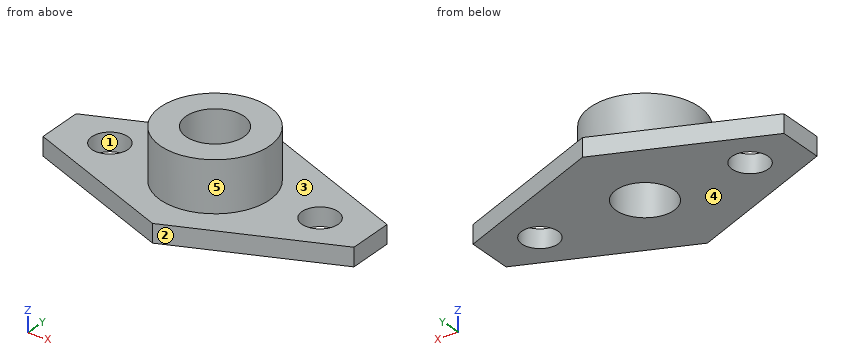
```python
from build123d import *

# Parameters (mm, degrees)
BOSS_EXTRUDE1_DEPTH     = 2.54
SKETCH1_4_R             = 7.560754729
BOSS_EXTRUDE2_DEPTH     = 9.525
CUT_EXTRUDE1_DEPTH      = 27.400295926
CUT_EXTRUDE1_DEPTH_BACK = 9.525
SKETCH1_8_R             = 4
SKETCH1_8_R_2           = 2.5


with BuildPart() as part:
    # Sketch1 → Boss-Extrude1 (new body)
    with BuildSketch(Plane.XY):
        Polygon((-21.5, 3.175), (0, 12), (21.5, 3.175), (21.5, 0), (21.5, -3.175), (0, -12), (-21.5, -3.175), align=None)
    extrude(amount=BOSS_EXTRUDE1_DEPTH)

    # Sketch1_4 → Boss-Extrude2 (add)
    with BuildSketch(Plane.XY):
        with Locations(Location((0, 0, 0), (0, 0, 180))):
            Circle(SKETCH1_4_R)
    extrude(amount=BOSS_EXTRUDE2_DEPTH)

    # Sketch1_8 → Cut-Extrude1 (cut, two sides: drawn at the far end of the back side and taken through both)
    with BuildSketch(Plane.XY.offset(-CUT_EXTRUDE1_DEPTH_BACK)):
        with Locations(Location((0, 0, 0), (0, 0, 180))):
            Circle(SKETCH1_8_R)
        with Locations(Location((14.530377365, 0, 0), (0, 0, 180))):
            Circle(SKETCH1_8_R_2)
        with Locations(Location((-14.530377365, 0, 0), (0, 0, 180))):
            Circle(SKETCH1_8_R_2)
    extrude(amount=CUT_EXTRUDE1_DEPTH + CUT_EXTRUDE1_DEPTH_BACK, mode=Mode.SUBTRACT)


solid = part.part
```
Input: part model. Units: mm. Frame: model coordinates. Face numbers are marked on the shaded views. A direction names the side the tool comes from. Round coordinates to 2 decimals unless told otherwise and drop trailing zeros. Loops run counter-clockwise (first coordinate to the right, second up) from the corner with the lowest first, then second, coordinate; pieces in that order, holes last. Notation, with made-up numbers: (77.25, -33.5) - (134.25, -33.5) arc R18 ccw to (134.25, -18.5) - close; hole circle Ø3 at (-6, 77). An arc over 180 degrees is marked (long way). One line per item, written item: value. Start each with the question number.
(1) Ray query, line 1 (X direction, y = -0.25, z = 5.75); line 2 (Y direction, x = 0, z = 4.5); line 3 (Z direction, x = 8.5, y = 6.25). Return the intervals inside material, ascending. Write a range as [from, to].
(2) Section C-C, the plane x = 16.5. Return loops of the section in (y, z).
(3) Section D-D, the plane x = -6. Return loops of the section in (y, z) (3 decimals).
(4) Section B-B, the plane y = 0. Return loops of the section in (x, z) (3 decimals).
(5) Access query for the marked faces 4 and 5. Directions: +Z, -Z, +X, -X, +Y, -Y. A direction counts if a zero-diameter tool reaches every point of the face in a straight line with its end or side. Return the directions, or none.
(6) Contact query for flat-ended pins moving along their axis: P1, Ø3, axis at x = 14.53, y = 0, coming from the +Z side; P2, Ø2, axis at x = 3.5, y = -3, coming from the -Z side; P3, Ø2, axis at x = 2.5, z = 7, coming from the -Y side; P4, Ø1, axis at y = -1.5, z = 6.5, coming from the -X side. Output: stop coordinate, or through.
(7) Section A-A, the plane z = 1. Return loops of the section in (x, y) (3 decimals), plus the area to 3 significant figures.
(8) Draft query along X for the marked faces 1, 2 and 3. Return one class per face: +X half, -X half, draft (parallel to the pull), parting line (faces both ways), or undercut.
Results below:
1. line 1: [-7.56, -3.99], [3.99, 7.56]
1. line 2: [-7.56, -4], [4, 7.56]
1. line 3: [0, 2.54]
2. outline: (-5.23, 0) - (-1.54, 0) - (-1.54, 2.54) - (-5.23, 2.54) - close; (1.54, 0) - (5.23, 0) - (5.23, 2.54) - (1.54, 2.54) - close
3. outline: (-9.537, 0) - (9.537, 0) - (9.537, 2.54) - (4.601, 2.54) - (4.601, 9.525) - (-4.601, 9.525) - (-4.601, 2.54) - (-9.537, 2.54) - close
4. outline: (-21.5, 0) - (-17.03, 0) - (-17.03, 2.54) - (-21.5, 2.54) - close; (-12.03, 0) - (-4, 0) - (-4, 9.525) - (-7.561, 9.525) - (-7.561, 2.54) - (-12.03, 2.54) - close; (4, 0) - (12.03, 0) - (12.03, 2.54) - (7.561, 2.54) - (7.561, 9.525) - (4, 9.525) - close; (17.03, 0) - (21.5, 0) - (21.5, 2.54) - (17.03, 2.54) - close
5. face 4: -Z, +X, -X, +Y, -Y
5. face 5: +Z
6. P1: through
6. P2: z = 0
6. P3: y = -7.41
6. P4: x = -7.49
7. outline: (-21.5, -3.175) - (0, -12) - (21.5, -3.175) - (21.5, 3.175) - (0, 12) - (-21.5, 3.175) - close; hole circle Ø5 at (-14.53, 0); hole circle Ø8 at (0, 0); hole circle Ø5 at (14.53, 0)
7. area: 563 mm^2
8. face 1: undercut
8. face 2: +X half
8. face 3: draft
